Verification items for this drawing (mm, ordinates from the low corner). A direction names the side the tool comes from. Coordinates: 2 decimals unless noted, no trailing zeros. Order: outer loops, then holes, each group sorted by start corner. A loop starts at its lowest first (then second) coordinate and runs counter-clockwise, first axis right, second up. Notation, with made-up numbers: M 51,46 L 104,46 A28 cw 104,66 Z; hole C 44,-1 d1. An arc over 180 degrees is marked long. Use CSV: the item, a comma, the result in double quotes. Start each with the question number.
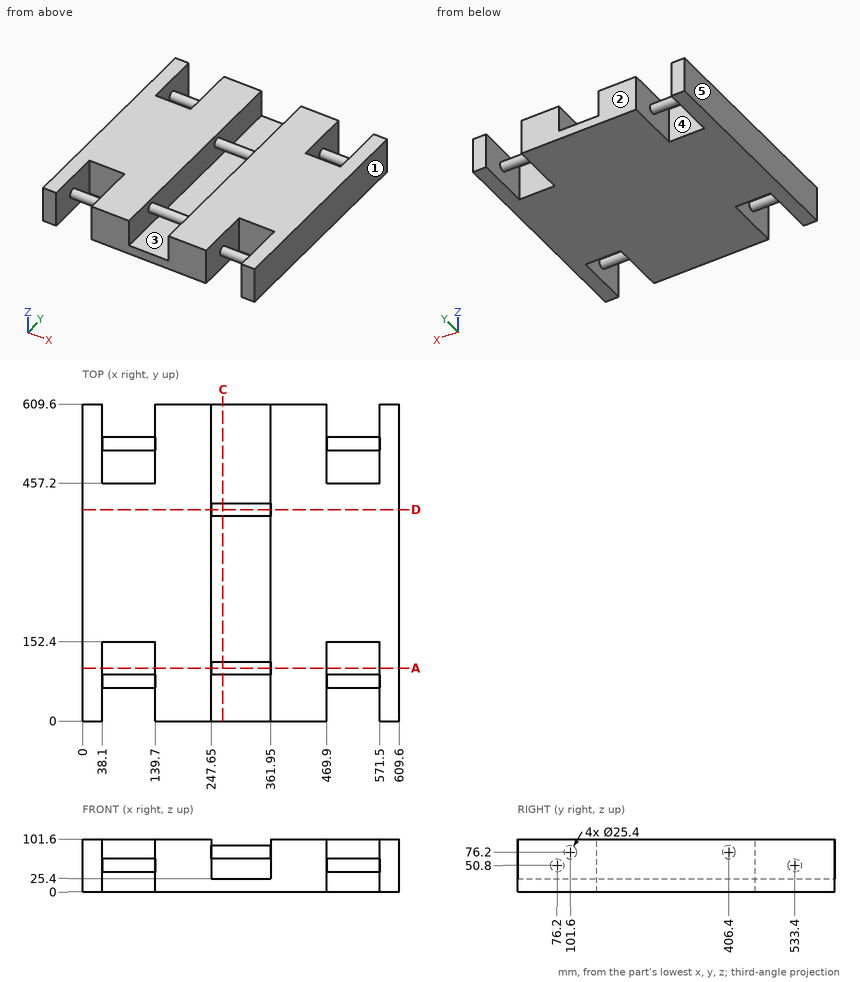
1) Section check D-D on y = 406.4. Record the boundary of the cut face in (x, z), then the cut area to 3 significant figures.
2) Section check C-C on x = 270. Record the boundary of the cut face in (y, z), then the cut area to 3 significant figures.
3) Gauge pin test, flat ends, axial feed: P1, Ø1.5, axis at x = 318, z = 86.5, coming from the +Y side; P2, Ø1.5, axis at x = 317.5, y = 93.5, coming from the +Z side; P3, Ø3, axis at x = 122, y = 527, coming from the +Z side. Record the tip position at first contact, or that the pin passes through.
4) Set-up check for the marked faces 4 and 5: record each of +Z, -Z, +X, -X, +Y, -Y from which the full face is reachable in a straight line by a thin tool's end or side.
5) Section check A-A on y = 101.6. Record the boundary of the cut face in (x, z).
6) Material ranges on line 1 along X through (y, z) = (37, 10.5); line 2 along X through (y, z) = (485, 43); line 3 along X through (y, z) = (369.5, 80), recorded low to high.
7) Draft check along X on the marked faces 1, 2 and 3. Enter one of: +X half, -X half, draft (parallel to the pull), parting line (faces both ways), or undercut.
Results are:
1,outline,"M 0,0 L 609.6,0 L 609.6,101.6 L 361.95,101.6 L 361.95,88.9 L 247.65,88.9 L 247.65,101.6 L 0,101.6 Z; hole M 247.65,25.4 L 361.95,25.4 L 361.95,63.5 L 247.65,63.5 Z"
1,area,"56,100 mm²"
2,outline,"M 0,0 L 609.6,0 L 609.6,25.4 L 0,25.4 Z; C 101.6,76.2 d25.4; C 406.4,76.2 d25.4"
2,area,"16,500 mm²"
3,P1,"stops at y = 414.77"
3,P2,"stops at z = 86.56"
3,P3,"stops at z = 62.52"
4,face 4,"+Z, -Z"
4,face 5,"+Z, -Z, -X, +Y, -Y"
5,outline,"M 0,0 L 38.1,0 L 38.1,101.6 L 0,101.6 Z; M 139.7,0 L 469.9,0 L 469.9,101.6 L 361.95,101.6 L 361.95,88.9 L 247.65,88.9 L 247.65,101.6 L 139.7,101.6 Z; M 571.5,0 L 609.6,0 L 609.6,101.6 L 571.5,101.6 Z; hole M 247.65,25.4 L 361.95,25.4 L 361.95,63.5 L 247.65,63.5 Z"
6,line 1,"x = 0 to 38.1, 139.7 to 469.9, 571.5 to 609.6"
6,line 2,"x = 0 to 38.1, 139.7 to 247.65, 361.95 to 469.9, 571.5 to 609.6"
6,line 3,"x = 0 to 247.65, 361.95 to 609.6"
7,face 1,"+X half"
7,face 2,"draft"
7,face 3,"undercut"
